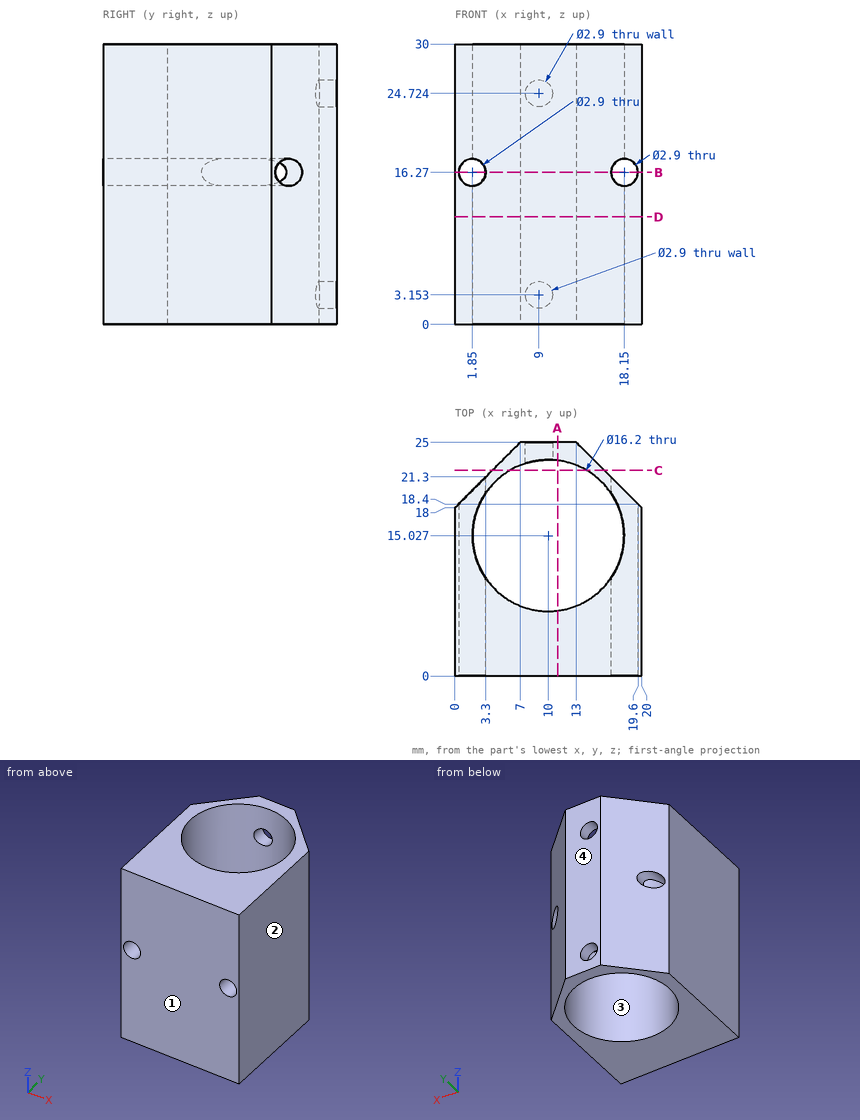
Here's the drawing with two shaded views (mm, measured from the low corner). I have some questions. Give positions to 0.01 mm unless a question says otherwise; leave off trailing zeros. Order: outer loops, then holes, each group sorted by start corner. A loop starts at its lowest first (then second) coordinate and runs counter-clockwise, first axis right, second up. Notation, with made-up numbers: M 22.25,1 L 74.25,1 A8 cw 74.25,15 Z; hole C 55.25,55.25 d3. An arc over 180 degrees is marked long. One line per item, written item: value.
1) We'd pull the mould along Y, two halves only. Please class the marked faces 1, 2, 3 and 4: released by +Y, released by -Y, zero draft, split by the parting line, or undercut.
Answer sheet:
face 1: released by -Y
face 2: zero draft
face 3: undercut
face 4: released by +Y
2) I want a section at D-D, the plane z = 11.5. List the corners of the cut face in (x, y) for me.
Answer sheet:
outline: M 0,0 L 20,0 L 20,18 L 13,25 L 7,25 L 0,18 Z; hole C 10,15.03 d16.2
3) I want a section at B-B, the plane z = 16.27. Count the separate pieces of the cut face and the enclosed holes in it, plus the area to 3 significant figures.
Answer sheet:
separate pieces: 4
enclosed holes: 0
area: 147 mm^2
4) Please list where these lines run through material, in increasing order: line 1 along Z through (x, y) = (18.15, 6.25); line 2 along X through (y, z) = (15, 7); line 3 along X through (y, z) = (6.25, 16) (1 decimal).
Answer sheet:
line 1: z = 0 to 14.82, 17.72 to 30
line 2: x = 0 to 1.9, 18.1 to 20
line 3: x = 0 to 0.4, 3.3 to 16.7, 19.6 to 20
5) For P1, Ø2.5, axis at x = 9, z = 24.72, coming from the +Y side (1 decimal); P2, Ø4.5, axis at x = 18.15, z = 16.27, coming from the -Y side, each with a flat end and sliding along its axis, tell me the tip position at first contact or that it passes through.
Answer sheet:
P1: stops at y = 7.2
P2: stops at y = 0
6) I want a section at C-C, the plane y = 22. List the corners of the cut face in (x, z) for me, plus the area to 3 significant figures.
Answer sheet:
outline: M 4,0 L 5.88,0 L 5.88,30 L 4,30 Z; M 14.12,0 L 16,0 L 16,30 L 14.12,30 Z
area: 113 mm^2
7) I want a section at A-A, the plane x = 11. List the corners of the cut face in (y, z) for me (1 decimal), plus the area to 3 significant figures.
Answer sheet:
outline: M 0,0 L 7,0 L 7,30 L 0,30 Z; M 23.1,0 L 25,0 L 25,30 L 23.1,30 Z
area: 268 mm^2
